Read the model definition and answer for the solid it produces. Units are mm, in the model's axes. A direction names the side the tool comes from. Coordinates: 2 decimals unless noted, no trailing zeros. Order: outer loops, then holes, each group sorted by start corner. A loop starts at its lowest first (then second) coordinate and runs counter-clockwise, first axis right, second up. Notation, with made-up numbers: (68.25, 72.25) - (88.25, 72.25) arc R17 cw to (88.25, 97.25) - close; hole circle Ø8 at (-33, 74). An arc over 180 degrees is marked (long way). Write item = value, one per line.
from build123d import *

# Parameters (mm, degrees)
F1_DEPTH = 15
F3_W     = 50
F3_H     = 50
F4_DEPTH = 30
F5_R     = 5
F6_DEPTH = 50


with BuildPart() as f1:
    # F0 (on Front) → F1 (new body)
    with BuildSketch(Plane.XZ):
        Polygon((0, 30), (0, 0), (30, 0), align=None)
    extrude(amount=-F1_DEPTH)

    # F3 (on offset) → F4 (join)
    with BuildSketch(Plane.XZ.offset(-15)):
        with Locations((25, 25)):
            Rectangle(F3_W, F3_H)
    extrude(amount=-F4_DEPTH)

    # F5 (on face) → F6 (join, through all)
    with BuildSketch(Plane.XY.offset(50)):
        with Locations((15, 30)):
            Circle(F5_R)
    extrude(amount=-F6_DEPTH)


solid = f1.part
1) Determine the mould class of faces 3 (the face through (25, 27, 0)), 4 (the face through (15, 7, 15)), 5 (the face through (0, 27, 25)) for opening direction X: pulls with the +X half, pulls with the -X half, needs draft (parallel to the pull), parting line crosses it, or undercut.
Returned:
face_3 = needs draft
face_4 = pulls with the +X half
face_5 = pulls with the -X half
2) The part is cut by section B-B (z = 12.5). Determine the outline of the cut face in (x, y), and give its area (3 significant figures).
Returned:
outline = (0, 0) - (17.5, 0) - (17.5, 15) - (50, 15) - (50, 45) - (0, 45) - close
area = 1,760 mm^2
3) The part is cut by section C-C (y = 6.5). Determine the outline of the cut face in (x, z), and give its area (3 significant figures).
Returned:
outline = (0, 0) - (30, 0) - (0, 30) - close
area = 450 mm^2
4) Straight lines are drawn through the part: line 1 along Y through (x, z) = (37.5, 29.5); line 2 along Z through (x, y) = (7, 14.5); line 3 along X through (y, z) = (5, 3.5). For each, find the intervals that lie inside material, in ascending order. Write a range as from..to.
Returned:
line_1 = 15..45
line_2 = 0..23
line_3 = 0..26.5
5) For faces 1 (the face through (30, 15, 31)), 2 (the face through (25, 45, 25)), determine the directions among +Z, -Z, +X, -X, +Y, -Y from which every point of the face is accessible in a straight line to the end or side of a thin tool.
Returned:
face_1 = +Z, +X, -Y
face_2 = +Z, -Z, +X, -X, +Y
6) A flat-ended cylindrical pin translates along its axis: pin 1 Ø10 at (x, z) = (44, 6.5) entering from -Y. Find the tip coordinate at first contact, or state that the pin passes through.
Returned:
pin_1 = 15
7) The part is cut by section A-A (x = 6). Determine the outline of the cut face in (y, z).
Returned:
outline = (0, 0) - (45, 0) - (45, 50) - (15, 50) - (15, 24) - (0, 24) - close
8) The part is cut by section D-D (x = 32.5). Determine the outline of the cut face in (y, z).
Returned:
outline = (15, 0) - (45, 0) - (45, 50) - (15, 50) - close
